from build123d import *

# Parameters (mm, degrees)
SKETCH1_W           = 520
SKETCH1_H           = 215
BOSS_EXTRUDE1_DEPTH = 10
SKETCH2_W           = 10.131829772
SKETCH2_H           = 5
CUT_EXTRUDE1_DEPTH  = 216
LPATTERN1_COUNT     = 31
LPATTERN1_PITCH     = 16.8


with BuildPart() as part:
    # Sketch1 → Boss-Extrude1 (new body)
    with BuildSketch(Plane(origin=(0, 0, 0), x_dir=(0, 0, -1), z_dir=(1, 0, 0))):
        Rectangle(SKETCH1_W, SKETCH1_H)
    extrude(amount=BOSS_EXTRUDE1_DEPTH)

    # Sketch2 → Cut-Extrude1 (cut, through all)
    with BuildSketch(Plane(origin=(0, 107.5, 0), x_dir=(1, 0, 0), z_dir=(0, 1, 0))):
        with Locations((10, -252.5)):
            Rectangle(SKETCH2_W, SKETCH2_H)
    cut_extrude1 = extrude(amount=-CUT_EXTRUDE1_DEPTH, mode=Mode.SUBTRACT)

    # LPattern1: Cut-Extrude1 ×31
    with Locations(*[(0, 0, -i * LPATTERN1_PITCH) for i in range(1, LPATTERN1_COUNT)]):
        add(cut_extrude1, mode=Mode.SUBTRACT)


solid = part.part
Here's how the part is built. I have some questions about the finished solid (model axes, mm). Give positions to 0.01 mm unless a question says otherwise; leave off trailing zeros. One line per item, written item: value.
Q1. If I drill on line 1 along X through (y, z) = (-20, 217), over which ranges is the centre line in solid material (lowest first)?
Answers follow:
line 1: 0 to 4.93
Q2. I'm going to push a flat-ended pin straight in: pin 1 Ø1.5 at (y, z) = (10.5, -99.5) entering from +X. Where does the tip first touch, or does it pass through?
Answers follow:
pin 1: x = 4.93
Q3. Suppose I cut it at A-A on x = 6.5. State how many separate pieces and enclosed holes the cut face has, then the cut area to 3 significant figures.
Answers follow:
separate pieces: 32
enclosed holes: 0
area: 78,500 mm^2
